Autodesk Inventor part; units mm, degrees
ref_plane "YZ Plane" through (0, 0, 0) normal (1, 0, 0) x (0, 1, 0)
ref_plane "XZ Plane" through (0, 0, 0) normal (0, 1, 0) x (-1, 0, 0)
ref_plane "XY Plane" through (0, 0, 0) normal (0, 0, 1) x (1, 0, 0)
sketch "Sketch1" plane through (0, 0, 0) normal (0, 0, 1) x (1, 0, 0)
  line L0 (0, 0) -> (25.4, 0)
  line L1 (25.4, 0) -> (25.4, 12.7)
  line L2 (25.4, 12.7) -> (0, 12.7)
  line L3 (0, 12.7) -> (0, 0)
  dimension "d0" = 25.4
  dimension "d1" = 12.7
extrude "Extrusion1" add sketch "Sketch1" along normal blind 12.7
sketch "Sketch2" plane through (0, 12.7, 0) normal (0, 1, 0) x (1, 0, 0)
  line L0 (5.398, -2.6368) -> (19.9399, -2.6368)
  line L1 (19.9399, -2.6368) -> (19.9399, -10.3739)
  line L2 (19.9399, -10.3739) -> (5.398, -10.3739)
  line L3 (5.398, -10.3739) -> (5.398, -2.6368)
extrude "Extrusion2" add sketch "Sketch2" along normal blind 2.54
sketch "Sketch3" plane through (5.398, 12.7, 10.3739) normal (0, 0, 1) x (1, 0, 0)
  line L0 (14.5419, 2.54) -> (0, 2.54)
  line L1 (0, 2.54) -> (6.9268, 1.1079)
  line L2 (6.9268, 1.1079) -> (14.5419, 2.54)
  point P0 (-5.398, -12.7)
extrude "Extrusion3" cut sketch "Sketch3" against normal blind 50.8
properties part number "Switch"
Geometry: final body of the model. Coordinates: model frame, mm. A direction names the side the tool comes from. Round coordinates to 2 decimals unless told otherwise and drop trailing zeros. Loops run counter-clockwise (first coordinate to the right, second up) from the corner with the lowest first, then second, coordinate; pieces in that order, holes last. Notation, with made-up numbers: (12.5, -7.5) -> (62.5, -7.5) arc R23 cw to (62.5, 7.5) -> close; hole circle Ø5 at (40.5, 48). An arc over 180 degrees is marked (long way). One line per question, with ' | ' between items. Start each with the question number.
1. Set-up query: faces 1 (the face through (12.6, 13.7, 2.637)), 2 (the face through (13, 6, 12.7)), 3 (the face through (12.8, 13.7, 10.374)). Return all of +Z, -Z, +X, -X, +Y, -Y with unobstructed straight access to the full face (end or side cutting, diameter ignored); none if empty.
2. Line query: line 1 along Z through (x, y) = (11.5, 13.5); line 2 along Y through (x, z) = (3.25, 8); line 3 along Y through (x, z) = (7, 8.5). Output: solid intervals per line, ascending. Write a range as [from, to].
3. Section C-C on x = 10.25. Output: boundary loops of the cut face in (y, z).
4. Section D-D on x = 20.5. Output: boundary loops of the cut face in (y, z).
5. Section B-B on y = 13. Output: boundary loops of the cut face in (x, z).
6. Contact query for flat-ended pins moving along their axis: pin 1 (2 mm diameter, centred on x = 16.5, z = 7.5, fed in from +Y); pin 2 (3 mm diameter, centred on y = 14.5, z = 6, fed in from -X); pin 3 (2 mm diameter, centred on x = 13.5, z = 9.5, fed in from +Y). Output: stop coordinate, or through.
7. Section A-A on z = 10. Output: boundary loops of the cut face in (x, y).
8. Mould query, pull axis X, two halves, no side actions, for faces 4 (the face through (8.813, 14.534, 6.56)), 5 (the face through (5.398, 14, 7)), 6 (the face through (16.079, 14.514, 6.56)), 7 (the face through (19.94, 14, 6)). Classes: pulls with the +X half, pulls with the -X half, needs draft (parallel to the pull), parting line crosses it, or undercut.
Returned:
1) face 1: -Z, +X, -X, +Y | face 2: +Z, +X, -X, +Y, -Y | face 3: +Z, +X, -X, +Y
2) line 1: z = [2.64, 10.37] | line 2: y = [0, 12.7] | line 3: y = [0, 14.91]
3) outline: (0, 0) -> (12.7, 0) -> (12.7, 2.64) -> (14.24, 2.64) -> (14.24, 10.37) -> (12.7, 10.37) -> (12.7, 12.7) -> (0, 12.7) -> close
4) outline: (0, 0) -> (12.7, 0) -> (12.7, 12.7) -> (0, 12.7) -> close
5) outline: (5.4, 2.64) -> (19.94, 2.64) -> (19.94, 10.37) -> (5.4, 10.37) -> close
6) pin 1: stops at y = 14.78 | pin 2: stops at x = 5.4 | pin 3: stops at y = 14.22
7) outline: (0, 0) -> (25.4, 0) -> (25.4, 12.7) -> (19.94, 12.7) -> (19.94, 15.24) -> (12.32, 13.81) -> (5.4, 15.24) -> (5.4, 12.7) -> (0, 12.7) -> close
8) face 4: undercut | face 5: pulls with the -X half | face 6: undercut | face 7: pulls with the +X half
